Autodesk Inventor part; units mm, degrees
ref_plane "YZ Plane" through (0, 0, 0) normal (1, 0, 0) x (0, 1, 0)
ref_plane "XZ Plane" through (0, 0, 0) normal (0, 1, 0) x (-1, 0, 0)
ref_plane "XY Plane" through (0, 0, 0) normal (0, 0, 1) x (1, 0, 0)
sketch "Sketch2" plane through (0, 0, 0) normal (0, 1, 0) x (-1, 0, 0)
  line L0 (-21.15, 21.15) -> (21.15, 21.15)
  line L1 (21.15, 21.15) -> (21.15, -21.15)
  line L2 (21.15, -21.15) -> (-21.15, -21.15)
  line L3 (-21.15, -21.15) -> (-21.15, 21.15)
  line L4 (-21.15, 21.15) -> (21.15, -21.15) construction
  line L5 (21.15, 21.15) -> (-21.15, -21.15) construction
  point P0 (0, 0)
  dimension "d0" = 42.3
  dimension "d1" = 42.3
extrude "Extrusion1" add sketch "Sketch2" along normal blind 28
sketch "Sketch3" plane through (0, 28, 0) normal (0, 1, 0) x (1, 0, 0)
  circle A0 centre (0, 0) radius 11
  dimension "d4" = 22
extrude "Extrusion2" add sketch "Sketch3" along normal blind 2
sketch "Sketch4" plane through (0, 28, 0) normal (0, 1, 0) x (1, 0, 0)
  line L0 (-24.8242, 0) -> (26.7617, 0) construction
  line L1 (0, -32.5742) -> (0, 40.8086) construction
  point P0 (0, 0)
  point P1 (-15.5, -15.5)
  point P2 (-15.5, 15.5)
  point P3 (15.5, -15.5)
  point P4 (15.5, 15.5)
  dimension "d7" = 15.5
  dimension "d8" = 15.5
  dimension "d9" = 0
  dimension "d10" = 0
  dimension "d11" = 26.7617
  dimension "d12" = 40.8086
  dimension "d13" = 32.5742
  dimension "d14" = 24.8242
hole "Hole1" at (-15.5, 28, 15.5) at (-15.5, 28, -15.5) at (15.5, 28, 15.5) at (15.5, 28, -15.5) direction (0, -1, 0) diameter 3 end through all
sketch "Sketch5" plane through (0, 30, 0) normal (0, 1, 0) x (1, 0, 0)
  circle A0 centre (0, 0) radius 2.5
  dimension "d22" = 5
extrude "Extrusion3" add sketch "Sketch5" along normal blind 24
sketch "Sketch6" plane through (0, 28, 0) normal (0, 1, 0) x (1, 0, 0)
  line L0 (-21.15, -21.15) -> (21.15, -21.15) construction
  line L1 (-21.15, 21.15) -> (-21.15, -21.15) construction
  line L2 (21.15, -21.15) -> (21.15, 21.15) construction
  line L3 (21.15, 21.15) -> (-21.15, 21.15) construction
  line L4 (-17.6145, -21.15) -> (-21.15, -17.6145)
  line L5 (-24, 0) -> (25, 0) construction
  line L6 (0, -28) -> (0, 33.5057) construction
  line L7 (-17.6145, 21.15) -> (-21.15, 17.6145)
  line L8 (17.6145, -21.15) -> (21.15, -17.6145)
  line L9 (17.6145, 21.15) -> (21.15, 17.6145)
  line L10 (-17.6145, -21.15) -> (-21.15, -21.15)
  line L11 (-21.15, -21.15) -> (-21.15, -17.6145)
  line L12 (-21.15, -21.15) -> (-21.15, 21.15)
  line L13 (-21.15, 21.15) -> (21.15, 21.15)
  line L14 (-17.6145, 21.15) -> (-21.15, 21.15)
  line L15 (-21.15, 21.15) -> (-21.15, 17.6145)
  line L16 (21.15, 21.15) -> (21.15, -21.15) construction
  line L17 (21.15, 17.6145) -> (21.15, 21.15)
  line L18 (21.15, 21.15) -> (17.6145, 21.15)
  line L19 (21.15, -21.15) -> (-21.15, -21.15)
  line L20 (17.6145, -21.15) -> (21.15, -21.15)
  line L21 (21.15, -21.15) -> (21.15, -17.6145)
  point P0 (0, 0)
  dimension "d25" = 5
  dimension "d33" = 3.5355
  dimension "d34" = 3.5355
  dimension "d35" = 3.5355
extrude "Extrusion4" cut sketch "Sketch6" against normal up to surface (28 mm away)
equation "\"d33\" = d34"
properties part number "Motor" material "Aluminum 6061"
Can you work these out from the model? Positions are in its coordinate system, mm. A direction names the side the tool comes from. Coordinates: 2 decimals unless noted, no trailing zeros. Loops run counter-clockwise (first coordinate to the right, second up) from the corner with the lowest first, then second, coordinate; pieces in that order, holes last. Notation, with made-up numbers: (83.25, -33.5) - (91.25, -33.5) arc R11 cw to (91.25, -25.5) - close; hole circle Ø6 at (-23.75, 58). An arc over 180 degrees is marked (long way). Answer as a JSON object with one key per item and string values. Group by question number.
Item 1: If we mould it in two halves opening along Z, with no side actions, what happens to faces 3 (the face through (-21.15, 14, 0)), 4 (the face through (15.43, 13.8, 14)), 5 (the face through (-2.38, 28.99, -10.74)), 6 (the face through (15.43, 13.8, -17))? For each: released by +Z, released by -Z, zero draft, split by the parting line, or undercut.
Item 2: If I drill on L1, parallel to X at y = 22.25, z = -15.5; L2, parallel to Y at x = 3, z = 14.5, over which ranges is the centre line in solid material (lowest first)? Write a range as from..to.
Item 3: If we section it at C-C (y = 16.5): List the corners of the cut face in (x, z) for me.
Item 4: If we section it at A-A (x = -15.5): List the corners of the cut face in (y, z) for me, plus the area to 3 significant figures.
Item 5: If we section it at B-B (z = 15.5): List the corners of the cut face in (x, y) for me.
Item 6: For pin 1 (1 mm diameter, centred on y = 35, z = 4, fed in from +X); pin 2 (3.5 mm diameter, centred on x = 15.5, z = 15.5, fed in from +Y); pin 3 (2 mm diameter, centred on x = 5.5, z = 0, fed in from +Y), each with a flat end and sliding along its axis, tell me the tip position at first contact or that it passes through.
Item 7: On a 3-axis mill with a long thin cutter (end or side, diameter ignored), from which of +Z, -Z, +X, -X, +Y, -Y can I reach the whole of each face in a straight line? I mean faces 1 (the face through (19.358, 14.196, -19.407)), 2 (the face through (-0.54, 41.83, -2.44)). Say none if no direction works.
Item 8: If we section it at D-D (z = 0): List the corners of the cut face in (x, y) for me.
Returned:
{
 "1": {"face 3": "zero draft", "face 4": "undercut", "face 5": "split by the parting line", "face 6": "undercut"},
 "2": {"L1": "x = -21.15..-17, -14..14, 17..21.15", "L2": "y = 0..28"},
 "3": {"outline": "(-21.15, -17.61) - (-17.61, -21.15) - (17.61, -21.15) - (21.15, -17.61) - (21.15, 17.61) - (17.61, 21.15) - (-17.61, 21.15) - (-21.15, 17.61) - close; hole circle Ø3 at (-15.5, -15.5); hole circle Ø3 at (-15.5, 15.5); hole circle Ø3 at (15.5, -15.5); hole circle Ø3 at (15.5, 15.5)"},
 "4": {"outline": "(0, -21.15) - (28, -21.15) - (28, -17) - (0, -17) - close; (0, -14) - (28, -14) - (28, 14) - (0, 14) - close; (0, 17) - (28, 17) - (28, 21.15) - (0, 21.15) - close", "area": "1,020 mm²"},
 "5": {"outline": "(-21.15, 0) - (-17, 0) - (-17, 28) - (-21.15, 28) - close; (-14, 0) - (14, 0) - (14, 28) - (-14, 28) - close; (17, 0) - (21.15, 0) - (21.15, 28) - (17, 28) - close"},
 "6": {"pin 1": "passes through", "pin 2": "stops at y = 28", "pin 3": "stops at y = 30"},
 "7": {"face 1": "-Z, +X, +Y, -Y", "face 2": "+Y"},
 "8": {"outline": "(-21.15, 0) - (21.15, 0) - (21.15, 28) - (11, 28) - (11, 30) - (2.5, 30) - (2.5, 54) - (-2.5, 54) - (-2.5, 30) - (-11, 30) - (-11, 28) - (-21.15, 28) - close"}
}
